Job drawing, mm, ordinate dimensions from the low corner. One solid piece. A direction names the side the tool comes from. Round coordinates to 2 decimals unless told otherwise and drop trailing zeros. Write each loop counter-clockwise with the first axis right and the second up, starting at its lowest first coordinate (ties: lowest second). Pieces come first, ordered by that corner, then holes.
1) Saw through at B-B (y = 22.25). Write the cut outline in (x, z) (1 decimal), plus the area to 3 significant figures.
2) Saw through at C-C (x = 31.5). Write the cut outline in (y, z) (1 decimal).
3) Saw through at A-A (z = 50). Write the cut outline in (x, y).
4) Saw through at D-D (y = 4.5). Write the cut outline in (x, z) (1 decimal), plus the area to 3 significant figures.
5) Flat gauge pins, fed straight in: pin 1 (7.5 mm diameter, centred on y = 14, z = 48, fed in from +X); pin 2 (12.5 mm diameter, centred on y = 15, z = 53, fed in from -X); pin 3 (12.5 mm diameter, centred on x = 46.5, y = 13, fed in from -Z); pin 4 (5 mm diameter, centred on x = 40, y = 4.5, fed in from +Z). Where does each tip first touch, or does it go through?
6) Pull direction Z, two halves, no side cores. Call the marked faces 1, 2 and 3: +Z half, -Z half, draft (parallel to the pull), parting line (faces both ways), or undercut.
7) Which spindle directions (+Z, -Z, +X, -X, +Y, -Y) get a long thin tool onto all of the face, cutting with end or side? Do the marked faces 4 and 5. Say none if no direction does.
8) Wall check: probe 1 along Z at (x, y) = (44, 22.25) (1 decimal); probe 2 along X at (y, z) = (22.5, 53); probe 3 along X at (y, z) = (17.75, 33). Give the ranges that are in metal, low to high.
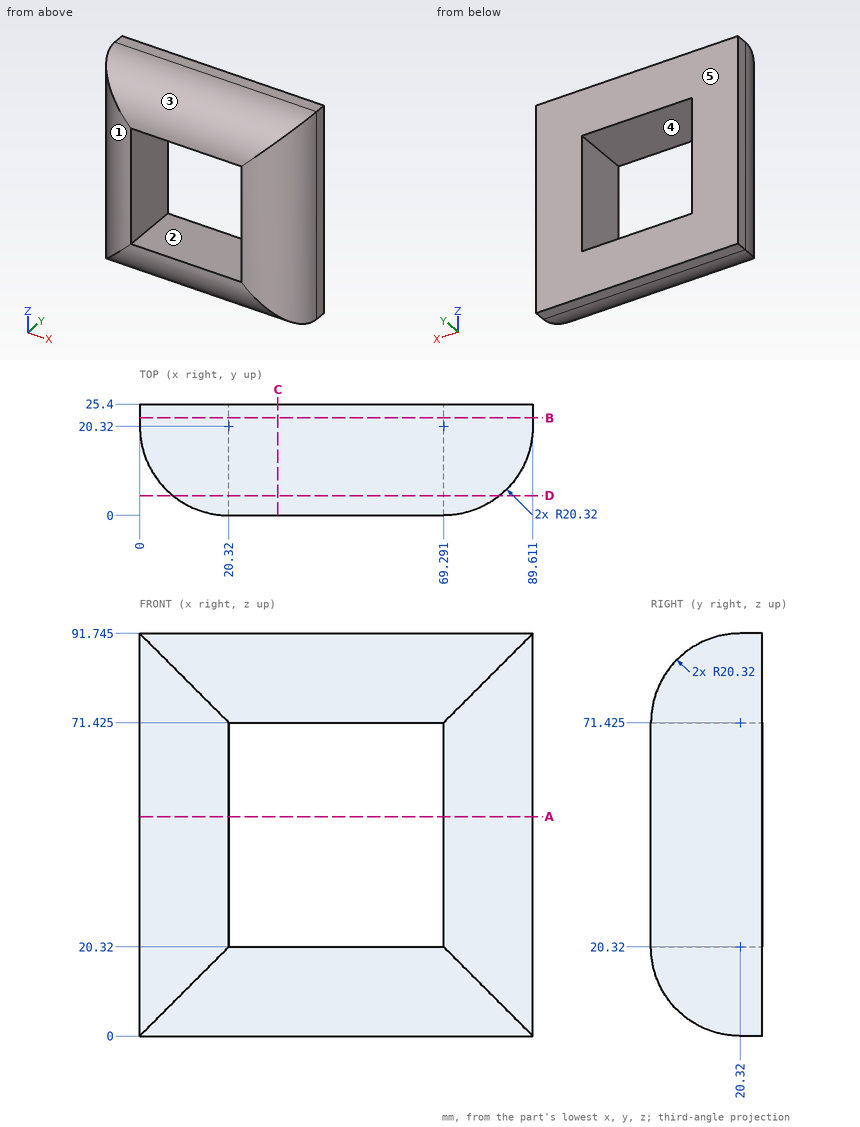
Evaluation:
1. outline: (0, 0) - (89.6, 0) - (89.6, 91.7) - (0, 91.7) - close; hole (20.3, 20.3) - (69.3, 20.3) - (69.3, 71.4) - (20.3, 71.4) - close
1. area: 5,720 mm2
2. outline: (0, 20.3) arc R20.3 ccw to (20.3, 0) - (25.4, 0) - (25.4, 20.3) - close; (0, 71.4) - (25.4, 71.4) - (25.4, 91.7) - (20.3, 91.7) arc R20.3 ccw to start
3. outline: (0, 20.32) arc R20.32 ccw to (20.32, 0) - (20.32, 25.4) - (0, 25.4) - close; (69.29, 0) arc R20.32 ccw to (89.61, 20.32) - (89.61, 25.4) - (69.29, 25.4) - close
4. outline: (7.6, 7.6) - (82, 7.6) - (82, 84.2) - (7.6, 84.2) - close; hole (20.3, 20.3) - (69.3, 20.3) - (69.3, 71.4) - (20.3, 71.4) - close
4. area: 3,200 mm2
5. pin 1: stops at x = 89.45
5. pin 2: stops at x = 0
5. pin 3: stops at z = 0.03
5. pin 4: stops at z = 86.77
6. face 1: draft
6. face 2: undercut
6. face 3: +Z half
7. face 4: +Y, -Y
7. face 5: +Z, -Z, +X, -X, +Y
8. probe 1: z = 0 to 20.3, 71.4 to 91.7
8. probe 2: x = 0 to 20.32, 69.29 to 89.61
8. probe 3: x = 0.16 to 20.32, 69.29 to 89.45
